Part print with two shaded views. Sizes in mm from the minimum x, y, z corner. Coordinates: 2 decimals unless noted, no trailing zeros. Write each loop counter-clockwise with the first axis right and the second up, starting at its lowest first coordinate (ties: lowest second). Pieces come first, ordered by that corner, then holes. Notation, with made-up numbers: (-37, 14.5) - (21, 14.5) arc R13 ccw to (21, 30.5) - close; hole circle Ø11 at (65, 20). An arc over 180 degrees is marked (long way). One line per question, with ' | ' between items. Start each with the question number.
1. Band-saw the part on B-B, the plane y = 7.5. Write the cut outline in (x, z).
2. Band-saw the part on C-C, the plane z = 0.3. Write the cut outline in (x, y), then the cut area to 3 significant figures.
3. Probe line 1 (Y direction, x = 56.5, z = 1.2); line 2 (Y direction, x = 34, z = 1.55); line 3 (X direction, y = 9, z = 0.8). List the from-to ranges inside material, lowest first.
4. Band-saw the part on A-A, the plane x = 34. Write the cut outline in (y, z).
5. Band-saw the part on D-D, the plane x = 11.5. Write the cut outline in (y, z), then the cut area to 3 significant figures.
6. Flat gauge pin, fed straight in: P1, Ø7, axis at x = 56.5, y = 52.5, coming from the -Z side. Where does the tip first touch, or does it go through?
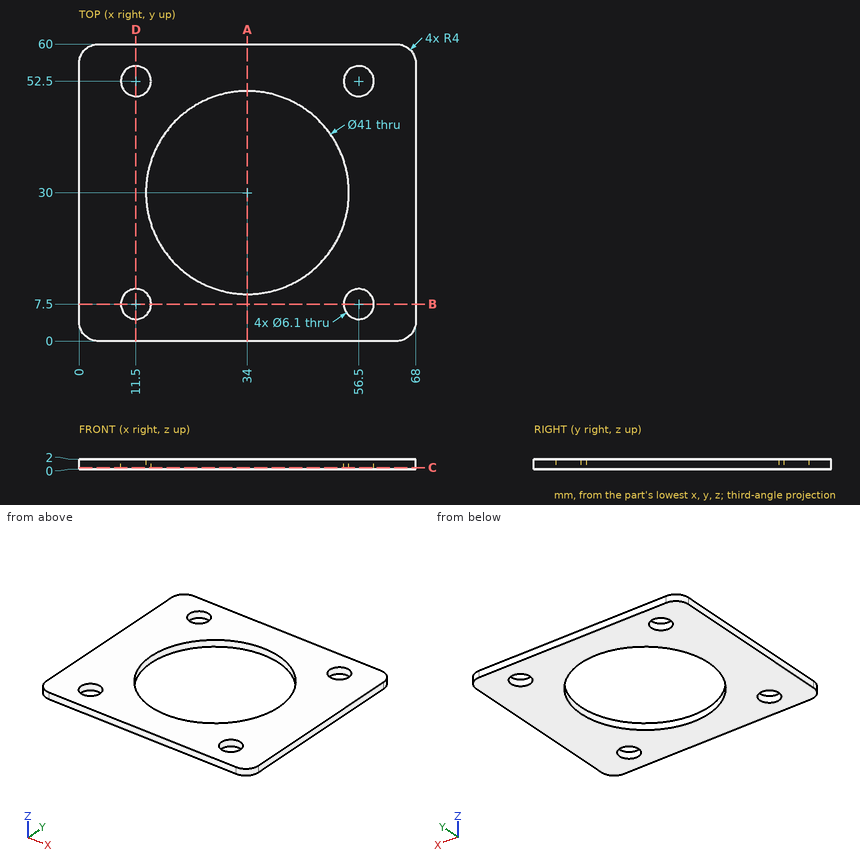
Filled in:
1) outline: (0, 0) - (8.45, 0) - (8.45, 2) - (0, 2) - close; (14.55, 0) - (53.45, 0) - (53.45, 2) - (14.55, 2) - close; (59.55, 0) - (68, 0) - (68, 2) - (59.55, 2) - close
2) outline: (0, 4) arc R4 ccw to (4, 0) - (64, 0) arc R4 ccw to (68, 4) - (68, 56) arc R4 ccw to (64, 60) - (4, 60) arc R4 ccw to (0, 56) - close; hole circle Ø6.1 at (11.5, 7.5); hole circle Ø6.1 at (11.5, 52.5); hole circle Ø41 at (34, 30); hole circle Ø6.1 at (56.5, 7.5); hole circle Ø6.1 at (56.5, 52.5) | area: 2,630 mm²
3) line 1: y = 0 to 4.45, 10.55 to 49.45, 55.55 to 60 | line 2: y = 0 to 9.5, 50.5 to 60 | line 3: x = 0 to 8.84, 14.16 to 53.84, 59.16 to 68
4) outline: (0, 0) - (9.5, 0) - (9.5, 2) - (0, 2) - close; (50.5, 0) - (60, 0) - (60, 2) - (50.5, 2) - close
5) outline: (0, 0) - (4.45, 0) - (4.45, 2) - (0, 2) - close; (10.55, 0) - (49.45, 0) - (49.45, 2) - (10.55, 2) - close; (55.55, 0) - (60, 0) - (60, 2) - (55.55, 2) - close | area: 95.6 mm²
6) P1: stops at z = 0
